Input: part model. Units: mm. Frame: model coordinates. Round coordinates to 2 decimals unless told otherwise and drop trailing zeros. Order: outer loops, then holes, each group sorted by start corner. A loop starts at its lowest first (then second) coordinate and runs counter-clockwise, first axis right, second up. Notation, with made-up numbers: (25.5, 25) - (69.5, 25) arc R26 ccw to (69.5, 62) - close; hole circle Ø10 at (-6.75, 42). An arc over 180 degrees is marked (long way). One line per item, written item: value. Start each with the question number.
from build123d import *

# Parameters (mm, degrees)
SKETCH1_R           = 55.88
BOSS_EXTRUDE1_DEPTH = 3.175
FILLET1_R           = 25.4


with BuildPart() as part:
    # Sketch1 → Boss-Extrude1 (new body)
    with BuildSketch(Plane(origin=(0, 0, 0), x_dir=(1, 0, 0), z_dir=(0, 1, 0))):
        with BuildLine():
            Line((87.63, 309.88), (436.88, 309.88))
            Line((436.88, 309.88), (436.88, 365.76))
            ThreePointArc((436.88, 365.76), (486.208175566, 440.496331963), (574.318959531, 424.518911361))
            Line((574.318959531, 424.518911361), (717.828959531, 287.358911361))
            ThreePointArc((717.828959531, 287.358911361), (742.95, 228.6), (717.828959531, 169.841088639))
            Line((717.828959531, 169.841088639), (574.318959531, 32.681088639))
            ThreePointArc((574.318959531, 32.681088639), (486.208175566, 16.703668037), (436.88, 91.44))
            Line((436.88, 91.44), (436.88, 147.32))
            Line((436.88, 147.32), (87.63, 147.32))
            ThreePointArc((87.63, 147.32), (6.35, 228.6), (87.63, 309.88))
        make_face()
        with Locations(Location((87.63, 228.6, 0), (0, 0, 270))):
            Circle(SKETCH1_R, mode=Mode.SUBTRACT)
        with Locations(Location((231.14, 228.6, 0), (0, 0, 270))):
            Circle(SKETCH1_R, mode=Mode.SUBTRACT)
        with Locations(Location((374.65, 228.6, 0), (0, 0, 270))):
            Circle(SKETCH1_R, mode=Mode.SUBTRACT)
        with Locations(Location((518.16, 228.6, 0), (0, 0, 270))):
            Circle(SKETCH1_R, mode=Mode.SUBTRACT)
        with Locations(Location((661.67, 228.6, 0), (0, 0, 270))):
            Circle(SKETCH1_R, mode=Mode.SUBTRACT)
        with Locations(Location((518.16, 365.76, 0), (0, 0, 270))):
            Circle(SKETCH1_R, mode=Mode.SUBTRACT)
        with Locations(Location((518.16, 91.44, 0), (0, 0, 270))):
            Circle(SKETCH1_R, mode=Mode.SUBTRACT)
    extrude(amount=BOSS_EXTRUDE1_DEPTH)

    # Fillet1
    fillet1_edges = [part.edges().sort_by_distance(p)[0] for p in [
        (436.88, 1.5875, -147.32),
        (436.88, 1.5875, -309.88),
    ]]
    fillet(fillet1_edges, radius=FILLET1_R)


solid = part.part
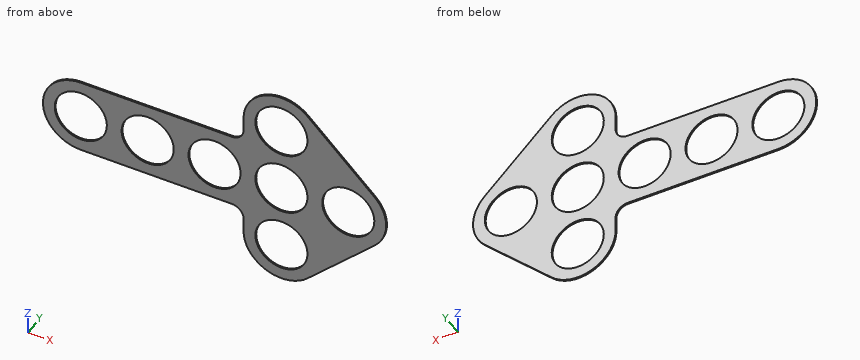
1. Section C-C (x = 231.14). Return the cut outline in (y, z) (3 decimals), then the cut area to 3 significant figures.
2. Line query: line 1 (X direction, y = 2.05, z = -228.6); line 2 (X direction, y = 2.75, z = -197.5); line 3 (X direction, y = 1, z = -134). Output: solid intervals per line, ascending. Write a range as from..to.
3. Section A-A (z = -228.6). Return the cut outline in (x, y) (3 decimals).
4. Section B-B (y = 1.6). Return the cut outline in (x, z).
5. Section D-D (x = 518.16). Return the cut outline in (y, z) (3 decimals).
6. Pin query (flat end, axial travel): pin 1 (1 mm diameter, centred on y = 0.5, z = -105, fed in from +X); pin 2 (1 mm diameter, centred on y = 1, z = -223, fed in from +X); pin 3 (1 mm diameter, centred on y = 0.5, z = -117, fed in from +X). Return the tip coordinate at first contact, or that it passes through.
Solved:
1. outline: (0, -309.88) - (3.175, -309.88) - (3.175, -284.48) - (0, -284.48) - close; (0, -172.72) - (3.175, -172.72) - (3.175, -147.32) - (0, -147.32) - close
1. area: 161 mm²
2. line 1: x = 6.35..31.75, 143.51..175.26, 287.02..318.77, 430.53..462.28, 574.04..605.79, 717.55..742.95
2. line 2: x = 12.54..41.2, 134.06..184.71, 277.57..328.22, 421.08..471.73, 564.59..615.24, 708.1..736.76
2. line 3: x = 433.82..481.95, 554.37..680.33
3. outline: (6.35, 0) - (31.75, 0) - (31.75, 3.175) - (6.35, 3.175) - close; (143.51, 0) - (175.26, 0) - (175.26, 3.175) - (143.51, 3.175) - close; (287.02, 0) - (318.77, 0) - (318.77, 3.175) - (287.02, 3.175) - close; (430.53, 0) - (462.28, 0) - (462.28, 3.175) - (430.53, 3.175) - close; (574.04, 0) - (605.79, 0) - (605.79, 3.175) - (574.04, 3.175) - close; (717.55, 0) - (742.95, 0) - (742.95, 3.175) - (717.55, 3.175) - close
4. outline: (87.63, -309.88) - (411.48, -309.88) arc R25.4 cw to (436.88, -335.28) - (436.88, -365.76) arc R81.28 ccw to (574.32, -424.52) - (717.83, -287.36) arc R81.28 ccw to (717.83, -169.84) - (574.32, -32.68) arc R81.28 ccw to (436.88, -91.44) - (436.88, -121.92) arc R25.4 cw to (411.48, -147.32) - (87.63, -147.32) arc R81.28 ccw to start; hole circle Ø111.76 at (87.63, -228.6); hole circle Ø111.76 at (231.14, -228.6); hole circle Ø111.76 at (374.65, -228.6); hole circle Ø111.76 at (518.16, -365.76); hole circle Ø111.76 at (518.16, -228.6); hole circle Ø111.76 at (518.16, -91.44); hole circle Ø111.76 at (661.67, -228.6)
5. outline: (0, -447.04) - (3.175, -447.04) - (3.175, -421.64) - (0, -421.64) - close; (0, -309.88) - (3.175, -309.88) - (3.175, -284.48) - (0, -284.48) - close; (0, -172.72) - (3.175, -172.72) - (3.175, -147.32) - (0, -147.32) - close; (0, -35.56) - (3.175, -35.56) - (3.175, -10.16) - (0, -10.16) - close
6. pin 1: stops at x = 650.51
6. pin 2: stops at x = 742.79
6. pin 3: stops at x = 663.06
